```python
from build123d import *

# Parameters (mm, degrees)
SKETCH1_W           = 45
SKETCH1_H           = 20
BOSS_EXTRUDE1_DEPTH = 1
SKETCH2_R           = 3.5
BOSS_EXTRUDE3_DEPTH = 13
SKETCH3_W           = 11.530514465
SKETCH3_H           = 3.932371985
BOSS_EXTRUDE4_DEPTH = 11
SKETCH4_W           = 10.630734434
SKETCH4_H           = 10.864010739
SKETCH4_W_2         = 12.863521917
SKETCH4_H_2         = 12.730221172
BOSS_EXTRUDE5_DEPTH = 6
SKETCH5_W           = 12.863521917
SKETCH5_H           = 12.730221172
BOSS_EXTRUDE6_DEPTH = 3
SKETCH6_W           = 6.198484655
SKETCH6_H           = 2.332763042
BOSS_EXTRUDE7_DEPTH = 3
SKETCH7_R           = 0.6
SKETCH7_R_2         = 2.133853082
CUT_EXTRUDE1_DEPTH  = 28.843311585


with BuildPart() as part:
    # Sketch1 → Boss-Extrude1 (new body)
    with BuildSketch(Plane(origin=(0, 0, 0), x_dir=(1, 0, 0), z_dir=(0, 1, 0))):
        Rectangle(SKETCH1_W, SKETCH1_H)
    extrude(amount=BOSS_EXTRUDE1_DEPTH)

    # Sketch2 → Boss-Extrude3 (add)
    with BuildSketch(Plane(origin=(0, 1, 0), x_dir=(1, 0, 0), z_dir=(0, 1, 0))):
        with Locations(Location((-17.029170207, 0, 0), (0, 0, 90))):
            Circle(SKETCH2_R)
        with Locations(Location((17.062495393, 0, 0), (0, 0, 90))):
            Circle(SKETCH2_R)
    extrude(amount=BOSS_EXTRUDE3_DEPTH)

    # Sketch3 → Boss-Extrude4 (add)
    with BuildSketch(Plane(origin=(0, 1, 0), x_dir=(1, 0, 0), z_dir=(0, 1, 0))):
        with Locations((4.898802389, 7.448179142)):
            Rectangle(SKETCH3_W, SKETCH3_H)
    extrude(amount=BOSS_EXTRUDE4_DEPTH)

    # Sketch4 → Boss-Extrude5 (add)
    with BuildSketch(Plane(origin=(0, 1, 0), x_dir=(1, 0, 0), z_dir=(0, 1, 0))):
        with Locations((-7.381528769, 4.482237559)):
            Rectangle(SKETCH4_W, SKETCH4_H)
        with Locations((5.565306115, -2.682677498)):
            Rectangle(SKETCH4_W_2, SKETCH4_H_2)
    extrude(amount=BOSS_EXTRUDE5_DEPTH)

    # Sketch5 → Boss-Extrude6 (add)
    with BuildSketch(Plane(origin=(0, 7, 0), x_dir=(1, 0, 0), z_dir=(0, 1, 0))):
        with Locations((5.565306115, -2.682677498)):
            Rectangle(SKETCH5_W, SKETCH5_H)
    extrude(amount=BOSS_EXTRUDE6_DEPTH)

    # Sketch6 → Boss-Extrude7 (add)
    with BuildSketch(Plane(origin=(0, 1, 0), x_dir=(1, 0, 0), z_dir=(0, 1, 0))):
        with Locations((-8.764524, -7.814756191)):
            Rectangle(SKETCH6_W, SKETCH6_H)
    extrude(amount=BOSS_EXTRUDE7_DEPTH)

    # Sketch7 → Cut-Extrude1 (cut, through all)
    with BuildSketch(Plane(origin=(0, 1, 0), x_dir=(1, 0, 0), z_dir=(0, 1, 0))):
        with Locations(Location((-21.528070359, 8.947812525, 0), (0, 0, 270))):
            Circle(SKETCH7_R)
        with Locations(Location((-21.528070359, -9.18108883, 0), (0, 0, 270))):
            Circle(SKETCH7_R)
        with Locations(Location((21.694696291, -9.18108883, 0), (0, 0, 270))):
            Circle(SKETCH7_R)
        with Locations(Location((21.694696291, 8.947812525, 0), (0, 0, 270))):
            Circle(SKETCH7_R)
        with Locations(Location((16.329341294, -7.314878396, 0), (0, 0, 270))):
            Circle(SKETCH7_R_2)
    extrude(amount=-CUT_EXTRUDE1_DEPTH, mode=Mode.SUBTRACT)


solid = part.part
```
Source: CAD feature listing. Evaluate the final solid. Frame: model axes, mm. A direction names the side the tool comes from. Round coordinates to 2 decimals unless told otherwise and drop trailing zeros. Loops run counter-clockwise (first coordinate to the right, second up) from the corner with the lowest first, then second, coordinate; pieces in that order, holes last. Notation, with made-up numbers: M 60.5,-15.5 L 90.5,-15.5 A25 ccw 90.5,17.5 Z; hole C 58.5,12 d5. An arc over 180 degrees is marked long. Use a Markdown table: item, result. Add a question column.
1. Contact query for flat-ended pins moving along their axis: pin 1 (1.4 mm diameter, centred on x = 21.69, z = 9.18, fed in from +Y); pin 2 (0.9 mm diameter, centred on x = -10, y = 3, fed in from -Z); pin 3 (3 mm diameter, centred on x = -17.5, y = 3, fed in from +Z). Output: stop coordinate, or through.
2. Cut plane C-C, the plane y = 2.25. Output: boundary loops of the cut face in (x, z).
3. Cut plane A-A, the plane y = 5. Output: boundary loops of the cut face in (x, z).
4. Pull-direction query (Z, two-part tool) for faces 1 (the flat face through (17, 14, 0)), 2 (the flat face through (-9, 2, 6.648)), 3 (the flat face through (5, 6, -9.414)); classes: +Z half, -Z half, draft (parallel to the pull), parting line (faces both ways), or undercut.
5. Cut plane B-B, the plane z = -6.25. Output: boundary loops of the cut face in (x, y).
6. Set-up query: faces 4 (the flat face through (-2.066, 4, -4)), 5 (the flat face through (-9, 4, 8)), 6 (the flat face through (5, 5, 9.048)), 7 (the cylindrical face through (-13.612, 7.409, 0.759)). Return all of +Z, -Z, +X, -X, +Y, -Y with unobstructed straight access to the full face (end or side cutting, diameter ignored); none if empty.
7. Cut plane D-D, the plane z = 7.75. Output: boundary loops of the cut face in (x, y).
8. Ray query, line 1 along X through (y, z) = (6.5, 0.25); line 2 along X through (y, z) = (1.5, -7.5); line 3 along Y through (x, z) = (-3.5, 4). Return the intervals inside material, ascending. Write a range as [from, to].
Solution:
| question | item | result |
|---|---|---|
| 1 | pin 1 | stops at y = 1 |
| 1 | pin 2 | stops at z = -9.91 |
| 1 | pin 3 | stops at z = 3.5 |
| 2 | outline | C -17.03,0 d7; M -12.7,-9.91 L -2.07,-9.91 L -2.07,0.95 L -12.7,0.95 Z; M -11.86,6.65 L -5.67,6.65 L -5.67,8.98 L -11.86,8.98 Z; M -0.87,-9.41 L 10.66,-9.41 L 10.66,-5.48 L -0.87,-5.48 Z; M -0.87,-3.68 L 12,-3.68 L 12,9.05 L -0.87,9.05 Z; C 17.06,0 d7 |
| 3 | outline | C -17.03,0 d7; M -12.7,-9.91 L -2.07,-9.91 L -2.07,0.95 L -12.7,0.95 Z; M -0.87,-9.41 L 10.66,-9.41 L 10.66,-5.48 L -0.87,-5.48 Z; M -0.87,-3.68 L 12,-3.68 L 12,9.05 L -0.87,9.05 Z; C 17.06,0 d7 |
| 4 | face 1 | draft |
| 4 | face 2 | undercut |
| 4 | face 3 | -Z half |
| 5 | outline | M -22.5,0 L 22.5,0 L 22.5,1 L 10.66,1 L 10.66,12 L -0.87,12 L -0.87,1 L -2.07,1 L -2.07,7 L -12.7,7 L -12.7,1 L -22.5,1 Z |
| 6 | face 4 | +Z, -Z, +Y |
| 6 | face 5 | +Z, -X, +Y |
| 6 | face 6 | +Z, +X, -X, +Y |
| 6 | face 7 | +Y |
| 7 | outline | M -22.5,0 L 14.24,0 L 14.24,1 L 12,1 L 12,10 L -0.87,10 L -0.87,1 L -5.67,1 L -5.67,4 L -11.86,4 L -11.86,1 L -22.5,1 Z; M 18.42,0 L 22.5,0 L 22.5,1 L 18.42,1 Z |
| 8 | line 1 | x = [-20.52, -13.54], [-12.7, -2.07], [-0.87, 12], [13.57, 20.55] |
| 8 | line 2 | x = [-12.7, -2.07], [-0.87, 10.66] |
| 8 | line 3 | y = [0, 1] |
